from build123d import *

# Parameters (mm, degrees)
F1_DEPTH       = 25
F2_R           = 1.2421542977
F3_DEPTH       = 5
F4_D           = 5
F4_CSINK_D     = 9
F4_CSINK_ANGLE = 90


with BuildPart() as f1:
    # F0 (on Front) → F1 (new body)
    with BuildSketch(Plane.XZ):
        Polygon((-8.5, -60), (-8.5, 60.2744125164), (-15, 60.2744125164), (-15, -69.7255874836), (15, -69.7255874836), (15, 60.2744125164), (8.5, 60.2744125164), (8.5, -60), align=None)
    extrude(amount=F1_DEPTH)

    # F2 (on Front) → F3 (join)
    with BuildSketch(Plane.XZ):
        Polygon((15, -70), (15, 0), (15, 60), (-15, 60), (-15, 0), (-15, -70), align=None)
        with Locations((0, -30)):
            Circle(F2_R, mode=Mode.SUBTRACT)
    extrude(amount=-F3_DEPTH)

    # F4 (through all)
    with Locations(Plane.XZ):
        with Locations((0, 30), (0, -30)):
            CounterSinkHole(F4_D / 2, F4_CSINK_D / 2, counter_sink_angle=F4_CSINK_ANGLE)


solid = f1.part
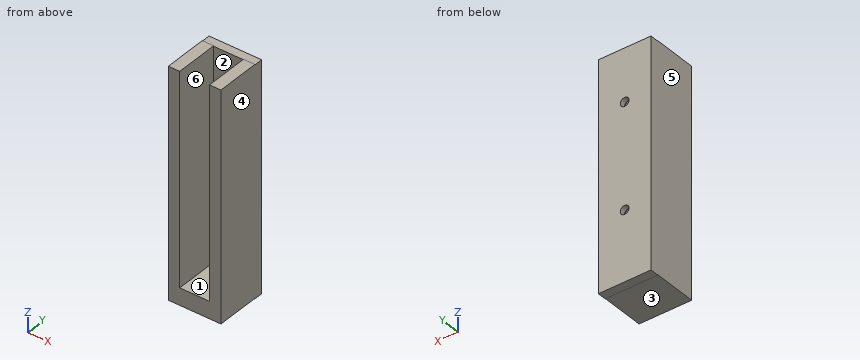
Geometry check sheet. Reference: the model listing, model coordinates, mm. Face numbers are marked on the shaded views. A direction names the side the tool comes from. Give positions to 0.01 mm unless a question says otherwise; leave off trailing zeros. Order: outer loops, then holes, each group sorted by start corner. A loop starts at its lowest first (then second) coordinate and runs counter-clockwise, first axis right, second up. Notation, with made-up numbers: M 39,39 L 94,39 A6 ccw 94,48 Z; hole C -3,-37.5 d10. An arc over 180 degrees is marked long. Use a Markdown table: item, result.
Item 1: Material ranges on line 1 along Z through (x, y) = (0, 3); line 2 along X through (y, z) = (2.8, 30); line 3 along X through (y, z) = (-4.5, -26), recorded low to high.
Answers follow:
| item | result |
|---|---|
| line 1 | z = -70 to -32.5, -27.5 to 27.5, 32.5 to 60 |
| line 2 | x = -15 to -2.5, 2.5 to 15 |
| line 3 | x = -15 to -8.5, 8.5 to 15 |
Item 2: Section check C-C (y = -6). Record the cut outline in (x, z), and give its area (3 significant figures).
Answers follow:
| item | result |
|---|---|
| outline | M -15,-69.73 L 15,-69.73 L 15,60.27 L 8.5,60.27 L 8.5,-60 L -8.5,-60 L -8.5,60.27 L -15,60.27 Z |
| area | 1,860 mm2 |
Item 3: Section check D-D (z = -48.5). Record the cut outline in (x, y), and give its area (3 significant figures).
Answers follow:
| item | result |
|---|---|
| outline | M -15,-25 L -8.5,-25 L -8.5,0 L 8.5,0 L 8.5,-25 L 15,-25 L 15,5 L -15,5 Z |
| area | 475 mm2 |
Item 4: Section check A-A (x = 0). Record the cut outline in (y, z), and give its area (3 significant figures).
Answers follow:
| item | result |
|---|---|
| outline | M -25,-69.73 L 0,-69.73 L 0,-70 L 5,-70 L 5,-32.5 L 2,-32.5 L 0,-34.5 L 0,-60 L -25,-60 Z; M 0,-25.5 L 2,-27.5 L 5,-27.5 L 5,27.5 L 2,27.5 L 0,25.5 Z; M 0,34.5 L 2,32.5 L 5,32.5 L 5,60 L 0,60 Z |
| area | 835 mm2 |
Item 5: Section check B-B (z = 30). Record the cut outline in (x, y), and give its area (3 significant figures).
Answers follow:
| item | result |
|---|---|
| outline | M -15,-25 L -8.5,-25 L -8.5,0 L -4.5,0 L -2.5,2 L -2.5,5 L -15,5 Z; M 2.5,2 L 4.5,0 L 8.5,0 L 8.5,-25 L 15,-25 L 15,5 L 2.5,5 Z |
| area | 446 mm2 |
Item 6: Depth check by flat-ended pin: P1, Ø6.5, axis at x = 0, z = -30, coming from the -Y side; P2, Ø1.5, axis at x = 11.5, y = -3.5, coming from the -Z side; P3, Ø13.5, axis at x = -3.5, z = -1, coming from the -Y side; P4, Ø4, axis at x = -6, z = 13.5, coming from the -Y side. Enter the tip coordinate at first touch or a pass-through.
Answers follow:
| item | result |
|---|---|
| P1 | stops at y = 1.25 |
| P2 | stops at z = -69.73 |
| P3 | stops at y = -25 |
| P4 | stops at y = 0 |
Item 7: Draft check along X on the marked faces 1, 2, 3 and 4. Enter one of: +X half, -X half, draft (parallel to the pull), parting line (faces both ways), or undercut.
Answers follow:
| item | result |
|---|---|
| face 1 | undercut |
| face 2 | undercut |
| face 3 | draft |
| face 4 | +X half |
Item 8: Tool access check on the marked faces 5 and 6. Record the directions out of +Z, -Z, +X, -X, +Y, -Y that give a thin tool (end or side, any length) a straight path to the whole face; none if there is none.
Answers follow:
| item | result |
|---|---|
| face 5 | +Z, -Z, -X, +Y, -Y |
| face 6 | +Z, -Y |
